For this review, take the finished solid that the model builds, in its own axes (mm). A direction names the side the tool comes from. Give positions to 0.01 mm unless a question says otherwise; leave off trailing zeros. Loops run counter-clockwise (first coordinate to the right, second up) from the corner with the lowest first, then second, coordinate; pieces in that order, holes last.
```python
from build123d import *

# Parameters (mm, degrees)
SKETCH1_R           = 2
BOSS_EXTRUDE1_DEPTH = 5
SKETCH3_R           = 2
BOSS_EXTRUDE2_DEPTH = 10


with BuildPart() as part:
    # Sketch1 → Boss-Extrude1 (new body)
    with BuildSketch(Plane(origin=(0, 0, 0), x_dir=(1, 0, 0), z_dir=(0, 1, 0))):
        with BuildLine():
            Line((0, 0), (25, 0))
            ThreePointArc((25, 0), (32.5, 7.5), (25, 15))
            Line((25, 15), (0, 15))
            ThreePointArc((0, 15), (-7.5, 7.5), (0, 0))
        make_face()
        with Locations((0, 7.5)):
            Circle(SKETCH1_R, mode=Mode.SUBTRACT)
        with Locations((25, 7.5)):
            Circle(SKETCH1_R, mode=Mode.SUBTRACT)
    extrude(amount=BOSS_EXTRUDE1_DEPTH)

    # Sketch3 → Boss-Extrude2 (add)
    with BuildSketch(Plane(origin=(0, 0, -15), x_dir=(-1, 0, 0), z_dir=(0, 0, -1))):
        with BuildLine():
            Line((-20, 5), (-5, 5))
            Line((-5, 5), (-5, 15))
            ThreePointArc((-5, 15), (-12.5, 22.5), (-20, 15))
            Line((-20, 15), (-20, 5))
        make_face()
        with Locations((-12.5, 15)):
            Circle(SKETCH3_R, mode=Mode.SUBTRACT)
    extrude(amount=-BOSS_EXTRUDE2_DEPTH)


solid = part.part
```
Item 1: Tool access review of faces 1 (the flat face through (20, 10, -10)), 2 (the flat face through (5, 10, -10)), 3 (the flat face through (13, 12, -5)): name each direction out of +Z, -Z, +X, -X, +Y, -Y from which nothing blocks a thin tool from reaching the whole face with its end or side.
Answer:
face 1: +Z, -Z, +X, +Y
face 2: +Z, -Z, -X, +Y
face 3: +Z, +X, -X, +Y
Item 2: Take a section at B-B on x = 12.5. Give the boundary of the cut face in (y, z).
Answer:
outline: (0, -15) - (13, -15) - (13, -5) - (5, -5) - (5, 0) - (0, 0) - close; (17, -15) - (22.5, -15) - (22.5, -5) - (17, -5) - close
Item 3: Take a section at D-D on z = -10.5. Give the boundary of the cut face in (x, y).
Answer:
outline: (-6.87, 0) - (31.87, 0) - (31.87, 5) - (20, 5) - (20, 15) arc R7.5 ccw to (5, 15) - (5, 5) - (-6.87, 5) - close; hole circle Ø4 at (12.5, 15)
Item 4: Take a section at A-A on z = -7.5. Give the boundary of the cut face in (x, y).
Answer:
outline: (-7.5, 0) - (-2, 0) - (-2, 5) - (-7.5, 5) - close; (2, 0) - (23, 0) - (23, 5) - (20, 5) - (20, 15) arc R7.5 ccw to (5, 15) - (5, 5) - (2, 5) - close; (27, 0) - (32.5, 0) - (32.5, 5) - (27, 5) - close; hole circle Ø4 at (12.5, 15)
Item 5: For L1, parallel to X at y = 2, z = -7.5; L2, parallel to Y at x = 12.5, z = -8.75; L3, parallel to Z at x = 0, y = 1.5, list the stretches that pass through material, from the lowest coordinate up.
Answer:
L1: x = -7.5 to -2, 2 to 23, 27 to 32.5
L2: y = 0 to 13, 17 to 22.5
L3: z = -15 to -9.5, -5.5 to 0
Item 6: The part is to be moulded in two halves that separate along X. For faces 4 (the cylindrical face through (12.34, 22.5, -10.07)), 5 (the cylindrical face through (12.76, 16.983, -10.07)), 6 (the flat face through (12, 2, 0)), say which applies: released by +X, released by -X, zero draft, split by the parting line, or undercut.
Answer:
face 4: split by the parting line
face 5: undercut
face 6: zero draft
Item 7: Take a section at C-C on y = 15.75. Give the boundary of the cut face in (x, z), and give its area (3 significant figures).
Answer:
outline: (5.04, -15) - (10.65, -15) - (10.65, -5) - (5.04, -5) - close; (14.35, -15) - (19.96, -15) - (19.96, -5) - (14.35, -5) - close
area: 112 mm2
Item 8: Clearance check with flat-ended pins moving along their axes: pin 1 Ø3 at (y, z) = (5, -2) entering from +X; pin 2 Ø1.5 at (x, z) = (7.5, -7) entering from +Y; pin 3 Ø2 at (x, y) = (4.5, 6.5) entering from -Z; pin 4 Ø4 at (x, z) = (-3, -5) entering from +Y. State where each tip first meets the part, or that it passes through.
Answer:
pin 1: stops at x = 31.34
pin 2: stops at y = 21.18
pin 3: stops at z = -15
pin 4: stops at y = 5
